Verification items for this drawing (mm, ordinates from the low corner). A direction names the side the tool comes from. Coordinates: 2 decimals unless noted, no trailing zeros. Write each loop counter-clockwise with the first axis right and the second up, starting at its lowest first coordinate (ties: lowest second). Pieces come first, ordered by that corner, then holes. Notation, with made-up numbers: (-29, 23.5) -> (-8, 23.5) arc R32 cw to (-8, 60.5) -> close; hole circle Ø9 at (-39, -13.75). An arc over 180 degrees is marked (long way). One line per question, with ' | ' between items.
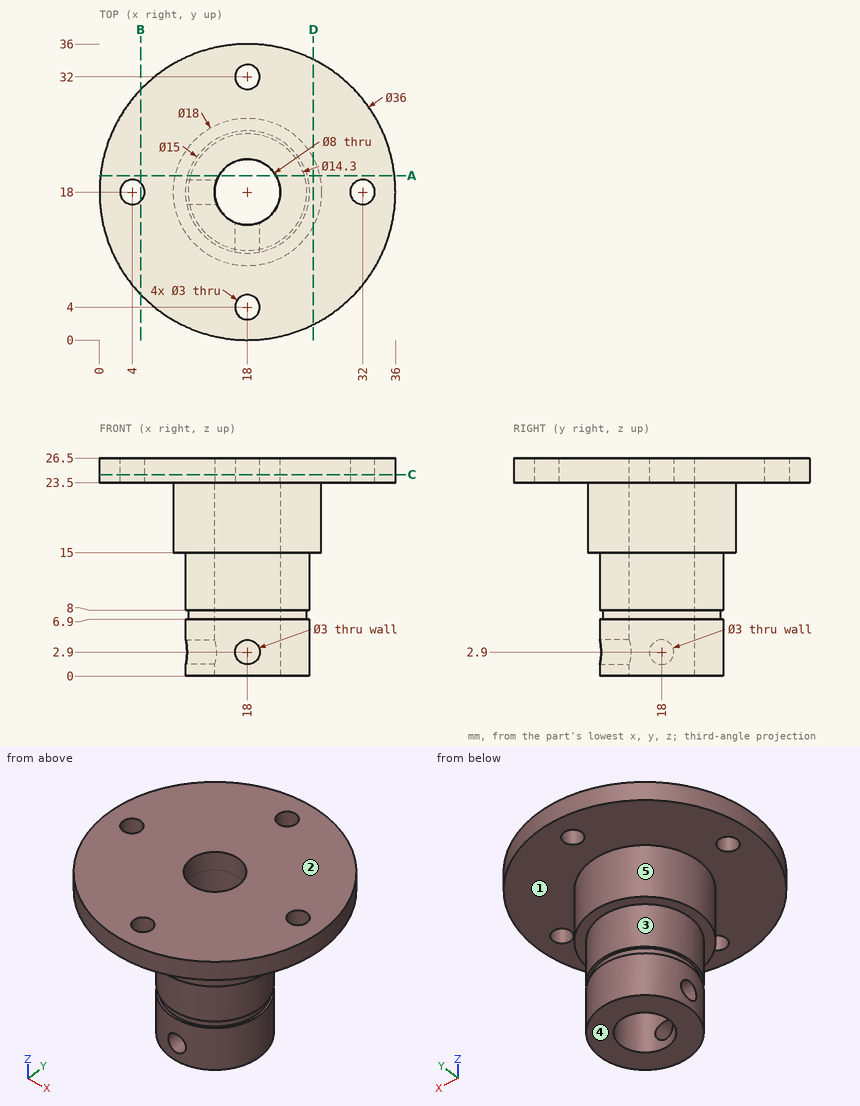
(1) Draft check along Z on the marked faces 1, 2 and 3. Enter one of: pulls with the +Z half, pulls with the -Z half, needs draft (parallel to the pull), parting line crosses it, or undercut.
Answers below:
face 1: pulls with the -Z half | face 2: pulls with the +Z half | face 3: needs draft
(2) Depth check by flat-ended pin: P1, Ø7.5, axis at x = 21, y = 15.5, coming from the -Z side; P2, Ø2.5, axis at y = 18, z = 2.9, coming from the -X side; P3, Ø2.5, axis at x = 18, z = 2.9, coming from the -Y side; P4, Ø2, axis at x = 24.5, z = 21, coming from the -Y side. Enter the tip coordinate at first touch or a pass-through.
Answers below:
P1: stops at z = 0 | P2: stops at x = 21.8 | P3: stops at y = 21.8 | P4: stops at y = 10.88
(3) Material ranges on line 1 (Y direction, x = 18, z = 24.3); line 2 (Z direction, x = 18, y = 13.35); line 3 (Z direction, x = 8.5, y = 12), recorded low to high.
Answers below:
line 1: y = 0 to 2.5, 5.5 to 14, 22 to 30.5, 33.5 to 36 | line 2: z = 0 to 1.4, 4.4 to 26.5 | line 3: z = 23.5 to 26.5
(4) Cross-section at A-A (y = 20). Record the cut outline in (x, z), plus the area to 3 significant figures.
Answers below:
outline: (0.11, 23.5) -> (9.23, 23.5) -> (9.23, 15) -> (10.77, 15) -> (10.77, 8) -> (11.14, 8) -> (11.14, 6.9) -> (10.77, 6.9) -> (10.77, 0) -> (14.54, 0) -> (14.54, 26.5) -> (0.11, 26.5) -> close; (21.46, 0) -> (25.23, 0) -> (25.23, 6.9) -> (24.86, 6.9) -> (24.86, 8) -> (25.23, 8) -> (25.23, 15) -> (26.77, 15) -> (26.77, 23.5) -> (35.89, 23.5) -> (35.89, 26.5) -> (21.46, 26.5) -> close | area: 289 mm²
(5) Tool access check on the marked faces 4 and 5. Record the directions out of +Z, -Z, +X, -X, +Y, -Y that give a thin tool (end or side, any length) a straight path to the whole face; none if there is none.
Answers below:
face 4: -Z, +X, -X, +Y, -Y | face 5: -Z
(6) Cross-section at B-B (x = 5). Record the cut outline in (y, z).
Answers below:
outline: (5.55, 23.5) -> (16.88, 23.5) -> (16.88, 26.5) -> (5.55, 26.5) -> close; (19.12, 23.5) -> (30.45, 23.5) -> (30.45, 26.5) -> (19.12, 26.5) -> close
(7) Cross-section at C-C (z = 24.5). Record the cut outline in (x, y).
Answers below:
outline: circle Ø36 at (18, 18); hole circle Ø3 at (4, 18); hole circle Ø8 at (18, 18); hole circle Ø3 at (18, 4); hole circle Ø3 at (18, 32); hole circle Ø3 at (32, 18)
(8) Cross-section at D-D (x = 26). Record the cut outline in (y, z).
Answers below:
outline: (1.88, 23.5) -> (13.88, 23.5) -> (13.88, 15) -> (22.12, 15) -> (22.12, 23.5) -> (34.12, 23.5) -> (34.12, 26.5) -> (1.88, 26.5) -> close
